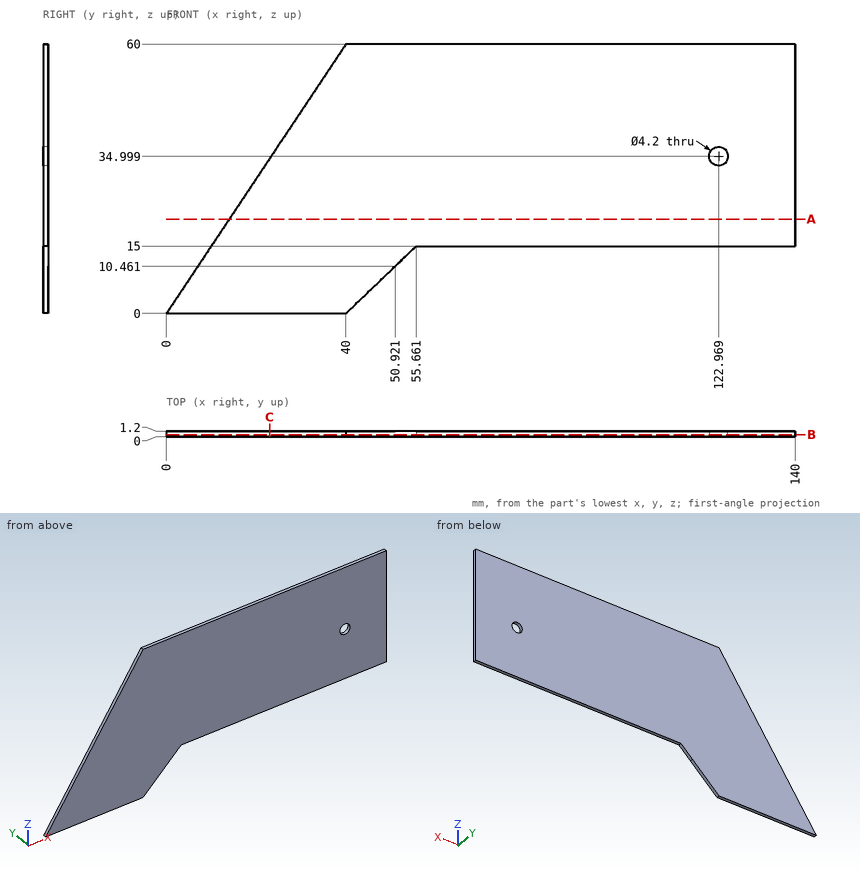
Study the drawing (mm; zero at the part's minimum x, y, z) and answer. Give positions to 0.01 mm unless a question says otherwise; leave off trailing zeros. Write each loop counter-clockwise with the first axis right and the second up, starting at its lowest first coordinate (ties: lowest second). Pieces come first, ordered by that corner, then holes. Notation, with made-up numbers: (6, 82.25) - (49, 82.25) arc R16 cw to (49, 99.25) - close; hole circle Ø11 at (-1.5, 48). An arc over 180 degrees is marked (long way). One line per question, with ' | ' between items. Start each with the question number.
1. Straight lines are drawn through the part: line 1 (Z direction, x = 57, y = 0.9); line 2 (X direction, y = 0.6, z = 33.5) (1 decimal); line 3 (X direction, y = 0.75, z = 36) (1 decimal). For each, find the intervals that lie inside material, in ascending order.
2. Section B-B, the plane y = 0.5 is taken. Determine the outline of the cut face in (x, z).
3. Section C-C, the plane x = 23 is taken. Determine the outline of the cut face in (y, z).
4. Section A-A, the plane z = 21 is taken. Determine the outline of the cut face in (x, y).
Result:
1) line 1: z = 15 to 60 | line 2: x = 22.3 to 121.5, 124.4 to 140 | line 3: x = 24 to 121.1, 124.8 to 140
2) outline: (0, 0) - (40, 0) - (55.66, 15) - (140, 15) - (140, 60) - (40, 60) - close; hole circle Ø4.2 at (122.97, 35)
3) outline: (0, 0) - (1.2, 0) - (1.2, 34.5) - (0, 34.5) - close
4) outline: (14, 0) - (140, 0) - (140, 1.2) - (14, 1.2) - close
